Input: part model. Units: mm. Frame: model coordinates. A direction names the side the tool comes from. Give positions to 0.01 mm unless a question says otherwise; leave off trailing zeros. Loops run counter-clockwise (first coordinate to the right, second up) from the corner with the lowest first, then second, coordinate; pieces in that order, holes last. Notation, with made-up numbers: (-21.75, 21) -> (1.25, 21) arc R26 ccw to (1.25, 39) -> close; hole circle Ø11 at (-8.5, 81.5). An arc over 180 degrees is marked (long way). Answer as a JSON object with one key per item and string values.
```python
from build123d import *

# Parameters (mm, degrees)
ESBO_O2_R          = 25.2
FLANGE_BASE1_DEPTH = 9.5
FILETE1_R          = 20


# Sheet-metal steps are written as plain solids
with BuildPart() as part:
    # Esboço2 → Flange-base1 (new body)
    with BuildSketch(Plane.XY):
        with BuildLine():
            Line((410.336115278, -12.808345835), (410.336115278, 47.191654165))
            Line((410.336115278, 47.191654165), (-410.063884722, 47.191654165))
            Line((-410.063884722, 47.191654165), (-410.063884722, -12.808345835))
            ThreePointArc((-410.063884722, -12.808345835), (-374.863884722, -48.008345835), (-339.663884722, -12.808345835))
            Line((-339.663884722, -12.808345835), (-260.063884722, -12.808345835))
            ThreePointArc((-260.063884722, -12.808345835), (-224.863884722, -48.008345835), (-189.663884722, -12.808345835))
            Line((-189.663884722, -12.808345835), (339.936115278, -12.808345835))
            ThreePointArc((339.936115278, -12.808345835), (375.136115278, -48.008345835), (410.336115278, -12.808345835))
        make_face()
        with Locations((375.136115278, -12.808345835)):
            Circle(ESBO_O2_R, mode=Mode.SUBTRACT)
        with Locations((-224.863884722, -12.808345835)):
            Circle(ESBO_O2_R, mode=Mode.SUBTRACT)
        with Locations((-374.863884722, -12.808345835)):
            Circle(ESBO_O2_R, mode=Mode.SUBTRACT)
    extrude(amount=-FLANGE_BASE1_DEPTH)

    # Filete1
    filete1_edges = [part.edges().sort_by_distance(p)[0] for p in [
        (339.936115278, -12.808345835, -4.75),
        (-189.663884722, -12.808345835, -4.75),
        (-260.063884722, -12.808345835, -4.75),
        (-339.663884722, -12.808345835, -4.75),
        (-410.063884722, 47.191654165, -4.75),
        (410.336115278, 47.191654165, -4.75),
    ]]
    fillet(filete1_edges, radius=FILETE1_R)


solid = part.part
```
Q1. Section B-B, the plane y = -5. Return the cut outline in (x, z), then the cut area to 3 significant figures.
Evaluation:
{"outline": "(-410.06, -9.5) -> (-398.82, -9.5) -> (-398.82, 0) -> (-410.06, 0) -> close; (-350.9, -9.5) -> (-248.82, -9.5) -> (-248.82, 0) -> (-350.9, 0) -> close; (-200.9, -9.5) -> (351.18, -9.5) -> (351.18, 0) -> (-200.9, 0) -> close; (399.1, -9.5) -> (410.34, -9.5) -> (410.34, 0) -> (399.1, 0) -> close", "area": "6,430 mm2"}
Q2. Pin query (flat end, axial travel): pin 1 (5 mm diameter, centred on x = -289.5, z = -5.5, fed in from -Y); pin 2 (5 mm diameter, centred on y = -23.5, z = -6, fed in from -X). Return the tip coordinate at first contact, or that it passes through.
Evaluation:
{"pin 1": "stops at y = -12.81", "pin 2": "stops at x = -409.1"}
Q3. Section C-C, the plane x = -212.5. Return the cut outline in (y, z), then the cut area to 3 significant figures.
Evaluation:
{"outline": "(-45.77, -9.5) -> (-34.77, -9.5) -> (-34.77, 0) -> (-45.77, 0) -> close; (9.15, -9.5) -> (47.19, -9.5) -> (47.19, 0) -> (9.15, 0) -> close", "area": "466 mm2"}
Q4. Section A-A, the plane z = -5.75. Return the cut outline in (x, y).
Evaluation:
{"outline": "(-410.06, -12.81) arc R35.2 ccw to (-342.06, -25.56) arc R20 cw to (-323.41, -12.81) -> (-276.31, -12.81) arc R20 cw to (-257.67, -25.56) arc R35.2 ccw to (-192.06, -25.56) arc R20 cw to (-173.41, -12.81) -> (323.69, -12.81) arc R20 cw to (342.33, -25.56) arc R35.2 ccw to (410.34, -12.81) -> (410.34, 27.19) arc R20 ccw to (390.34, 47.19) -> (-390.06, 47.19) arc R20 ccw to (-410.06, 27.19) -> close; hole circle Ø50.4 at (-374.86, -12.81); hole circle Ø50.4 at (-224.86, -12.81); hole circle Ø50.4 at (375.14, -12.81)"}
Q5. Draft query along Y for faces 3 (the flat face through (-6, 11, -9.5)), 4 (the cylindrical face through (-250.04, -11.7, -4.68)), 5 (the cylindrical face through (335.12, -16.4, -4.82)). Return one class per face: +Y half, -Y half, draft (parallel to the pull), parting line (faces both ways), or undercut.
Evaluation:
{"face 3": "draft", "face 4": "undercut", "face 5": "-Y half"}
Q6. Access query for faces 1 (the cylindrical face through (-334.85, -16.4, -4.82)), 2 (the cylindrical face through (-404.05, 41.49, -4.82)). Directions: +Z, -Z, +X, -X, +Y, -Y. A direction counts if a zero-diameter tool reaches every point of the face in a straight line with its end or side. Return the directions, or none.
Evaluation:
{"face 1": "+Z, -Z, -Y", "face 2": "+Z, -Z, -X, +Y"}
Q7. Section D-D, the plane x = -99.5. Return the cut outline in (y, z), then the cut area to 3 significant figures.
Evaluation:
{"outline": "(-12.81, -9.5) -> (47.19, -9.5) -> (47.19, 0) -> (-12.81, 0) -> close", "area": "570 mm2"}
Q8. Ray query, line 1 along X through (y, z) = (-7.5, -7.25); line 2 along X through (y, z) = (-18.5, -2.25); line 3 along Y through (x, z) = (278.5, -4.5). Return the intervals inside material, ascending.
Evaluation:
{"line 1": "x = -410.06 to -399.5, -350.23 to -249.5, -200.23 to 350.5, 399.77 to 410.34", "line 2": "x = -409.6 to -399.41, -350.32 to -337.39, -262.34 to -249.41, -200.32 to -187.39, 337.66 to 350.59, 399.68 to 409.87", "line 3": "y = -12.81 to 47.19"}
